Verification items for the finished model (mm, model axes). A direction names the side the tool comes from. Give positions to 0.01 mm unless a question says otherwise; leave off trailing zeros. Order: outer loops, then holes, each group sorted by start corner. A loop starts at its lowest first (then second) coordinate and runs counter-clockwise, first axis right, second up.
from build123d import *

# Parameters (mm, degrees)
BOSS_EXTRUDE1_DEPTH = 14.224
SKETCH2_W           = 10.16
SKETCH2_H           = 14.224
BOSS_EXTRUDE2_DEPTH = 7.112
SKETCH3_W           = 10.16
SKETCH3_H           = 7.112
REVOLVE2_ANGLE      = 180
CUT_EXTRUDE2_REACH  = 37.062
SKETCH5_R           = 2.032
BOSS_EXTRUDE4_DEPTH = 10.16
SKETCH8_R           = 2.286
CUT_EXTRUDE3_DEPTH  = 5.08


with BuildPart() as part:
    # Sketch1 → Boss-Extrude1 (new body)
    with BuildSketch(Plane(origin=(0, 0, 0), x_dir=(1, 0, 0), z_dir=(0, 1, 0))):
        Polygon((-6.487826296, -4.699), (6.487826296, -4.699), (10.16, -2.102598059), (18.587251519, -2.102598059), (18.587251519, -4.642598059), (10.967251519, -4.642598059), (7.295077814, -7.239), (-7.295077814, -7.239), (-12.7, -3.417462245), (-12.7, 3.417462245), (-7.295077814, 7.239), (7.295077814, 7.239), (10.967251519, 4.642598059), (18.587251519, 4.642598059), (18.587251519, 2.102598059), (10.16, 2.102598059), (6.487826296, 4.699), (-6.487826296, 4.699), (-10.16, 2.102598059), (-10.16, -2.102598059), align=None)
    extrude(amount=BOSS_EXTRUDE1_DEPTH)

    # Sketch2 → Boss-Extrude2 (add)
    with BuildSketch(Plane.XY.offset(7.239)):
        with Locations((0, 7.112)):
            Rectangle(SKETCH2_W, SKETCH2_H)
    extrude(amount=BOSS_EXTRUDE2_DEPTH)

    # Sketch3 → Revolve2 (revolve)
    with BuildSketch(Plane.XY.offset(14.351)):
        with Locations((0, 10.668)):
            Rectangle(SKETCH3_W, SKETCH3_H)
    revolve(axis=Axis((-5.08, 7.112, 14.351), (1, 0, 0)), revolution_arc=REVOLVE2_ANGLE)

    # Cut-Extrude2: up to this face of the body (flat: up to its plane)
    cut_extrude2_end = Plane(part.part.faces().sort_by_distance((14.777251519, 7.112, 4.642598059))[0])
    # Sketch5 → Cut-Extrude2 (cut, up to the picked face)
    with BuildSketch(Plane(origin=(0, 0, -4.642598059), x_dir=(-1, 0, 0), z_dir=(0, 0, -1)), mode=Mode.PRIVATE) as cut_extrude2_sk1:
        with Locations((-14.777251519, 7.112)):
            Circle(SKETCH5_R)
    cut_extrude2_tool1 = split(extrude(cut_extrude2_sk1.sketch, amount=-CUT_EXTRUDE2_REACH, mode=Mode.PRIVATE), bisect_by=cut_extrude2_end, keep=Keep.BOTH, mode=Mode.PRIVATE)
    add(cut_extrude2_tool1.solids().sort_by(Axis((14.777252, 7.112, -4.642598), (0, 0, 1)))[0], mode=Mode.SUBTRACT)

    # Sketch7 → Boss-Extrude4 (add)
    with BuildSketch(Plane(origin=(5.08, 0, 0), x_dir=(0, 0, -1), z_dir=(1, 0, 0))):
        Polygon((-27.259989759, -13.003831416), (-36.402849284, -2.10779573), (-37.831520464, -0.405171719), (-29.054109682, 6.959950431), (-27.625438502, 5.25732642), (-18.891073315, 12.586329027), (-9.748213789, 1.690293341), align=None)
        Polygon((-27.421266886, -9.409111436), (-32.890746657, -2.890839269), (-25.788748625, 3.06844466), (-20.319268854, -3.449827506), align=None, mode=Mode.SUBTRACT)
    extrude(amount=-BOSS_EXTRUDE4_DEPTH)

    # Sketch8 → Cut-Extrude3 (cut)
    with BuildSketch(Plane(origin=(0, 18.390622806, 15.431564813), x_dir=(1, 0, 0), z_dir=(0, 0.7660444431189808, 0.642787609686536))):
        with Locations(Location((0, -23.512017379, 0), (0, 0, 270))):
            Circle(SKETCH8_R)
    extrude(amount=-CUT_EXTRUDE3_DEPTH, mode=Mode.SUBTRACT)


solid = part.part
(1) Section check D-D, the plane z = 26.5. Enter the section's corners in (x, y), then the cut area to 3 significant figures.
Solved:
outline: (-5.08, -12.37) - (5.08, -12.37) - (5.08, -8.64) - (-5.08, -8.64) - close; (-5.08, 2.47) - (5.08, 2.47) - (5.08, 6.2) - (-5.08, 6.2) - close
area: 75.8 mm2
(2) Go/stop test with flat-tipped pins: pin 1 (5.5 mm diameter, centred on x = 2, z = 2.5, fed in from -Y); pin 2 (1.8 mm diameter, centred on x = 6.5, y = 4, fed in from +Z); pin 3 (2 mm diameter, centred on y = 3, z = 18, fed in from -X); pin 4 (3.5 mm diameter, centred on x = 14.78, y = 7.11, fed in from -Z). Record where each tip stops, or that it passes through.
Solved:
pin 1: stops at y = 0
pin 2: stops at z = 7.24
pin 3: stops at x = -5.08
pin 4: passes through
(3) Release check for a two-part mould opening along Z. For faces 6 (the flat face through (17, 9, 4.643)), 7 (the flat face through (18.587, 7, 3)), 8 (the flat face through (-8.35, 7.01, 3.38)) record: pulls with the +Z half, pulls with the -Z half, needs draft (parallel to the pull), parting line crosses it, or undercut.
Solved:
face 6: pulls with the +Z half
face 7: needs draft
face 8: undercut
(4) Section check A-A, the plane x = 4. Enter the section's corners in (y, z), then the cut area to 3 significant figures.
Solved:
outline: (-13, 27.26) - (0, 11.76) - (0, 4.7) - (14.22, 4.7) - (14.22, 14.35) arc R7.11 ccw to (12.53, 18.95) - (5.26, 27.63) - (6.96, 29.05) - (-0.41, 37.83) - close; (0, -7.24) - (14.22, -7.24) - (14.22, -4.7) - (0, -4.7) - close; hole (-9.41, 27.42) - (-3.45, 20.32) - (3.07, 25.79) - (-2.89, 32.89) - close
area: 444 mm2
(5) Set-up check for faces 1 (the flat face through (0.071, 8.845, 23.35)), 2 (the flat face through (-5.08, 4, 19)), 3 (the flat face through (0, 0, 6)), 4 (the flat face through (0, 7, 4.699)), 5 (the flat face through (13, 9, 2.103)): record each of +Z, -Z, +X, -X, +Y, -Y from which the full face is reachable in a straight line by a thin tool's end or side.
Solved:
face 1: +X, -X, +Y
face 2: +Z, -X, +Y, -Y
face 3: -Z, +X, -X, -Y
face 4: +Y, -Y
face 5: +X, +Y, -Y
(6) Section check B-B, the plane z = 4. Enter the section's corners in (x, y).
Solved:
outline: (-11.88, 0) - (-7.48, 0) - (-7.48, 14.22) - (-11.88, 14.22) - close; (7.48, 0) - (18.59, 0) - (18.59, 14.22) - (7.48, 14.22) - close; hole circle Ø4.06 at (14.78, 7.11)
(7) Section check C-C, the plane y = 8. Give the number of separate pieces and of enclosed holes in the cut face, then the cut area to 3 significant figures.
Solved:
separate pieces: 3
enclosed holes: 0
area: 331 mm2
(8) Scan lines: line 1 (Z direction, x = 0.5, y = 5.5); line 2 (Z direction, x = -1.5, y = 6.5); line 3 (X direction, y = 9, z = -0.5). Record each from-to range of solid material in increasing order.
Solved:
line 1: z = -7.24 to -4.7, 4.7 to 27.34, 27.83 to 30.79
line 2: z = -7.24 to -4.7, 4.7 to 26.14, 28.67 to 29.6
line 3: x = -12.7 to -10.16
